Source: CAD feature listing. Evaluate the final solid. Frame: model axes, mm. Face numbers are marked on the shaded views. Round coordinates to 2 decimals unless told otherwise and drop trailing zeros. Loops run counter-clockwise (first coordinate to the right, second up) from the corner with the lowest first, then second, coordinate; pieces in that order, holes last. Notation, with made-up numbers: M -33.5,-22.5 L -1.5,-22.5 A6 cw -1.5,-18.5 Z; hole C -21,-15 d7. An arc over 180 degrees is marked long. Answer as CSV lines item,"result". Start each with the question number.
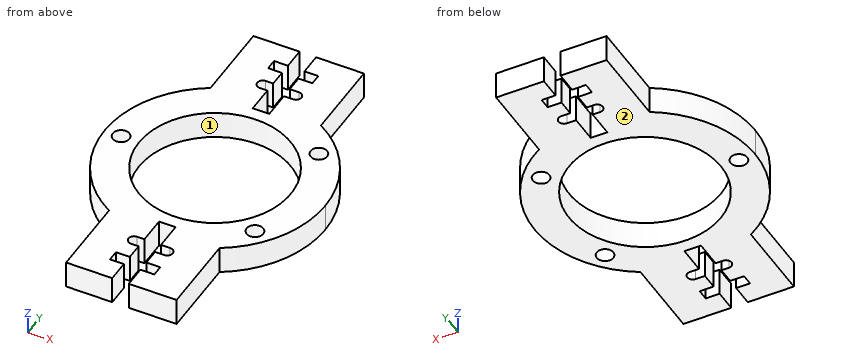
```python
from build123d import *
from build123d.topology import SkipClean

# Parameters (mm, degrees)
SKETCH1_R           = 1.5
BOSS_EXTRUDE1_DEPTH = 5


with BuildPart() as part:
    # Sketch1 → Boss-Extrude1 (new body)
    with BuildSketch(Plane(origin=(0, 0, 0), x_dir=(-0.9999998655639977, -0.000518528674721734, 0), z_dir=(0, 0, 1))):
        with BuildLine():
            Line((20, 0), (18.5, 0))
            ThreePointArc((18.5, 0), (17, -1.5), (15.5, 0))
            Line((15.5, 0), (13.75, 0))
            ThreePointArc((13.75, 0), (0, -13.75), (-13.75, 0))
            Line((-13.75, 0), (-20, 0))
            ThreePointArc((-20, 0), (-17.320508076, -10), (-10, -17.320508076))
            Line((-10, -17.320508076), (-10, -32))
            Line((-10, -32), (-1.347069158, -32))
            Line((-1.347069158, -32), (-1.347069158, -28.031929013))
            Line((-1.347069158, -28.031929013), (-3.861161574, -28.031929013))
            Line((-3.861161574, -28.031929013), (-3.861161574, -26))
            Line((-3.861161574, -26), (-1.347069158, -26))
            Line((-1.347069158, -26), (-1.347069158, -23))
            Line((-1.347069158, -23), (-3, -23))
            ThreePointArc((-3, -23), (-4, -22), (-3, -21))
            Line((-3, -21), (-1.347069158, -21))
            Line((-1.347069158, -21), (-1.347069158, -16))
            Line((-1.347069158, -16), (1.652930842, -16))
            Line((1.652930842, -16), (1.652930842, -21))
            Line((1.652930842, -21), (3, -21))
            ThreePointArc((3, -21), (4, -22), (3, -23))
            Line((3, -23), (1.652930842, -23))
            Line((1.652930842, -23), (1.652930842, -26))
            Line((1.652930842, -26), (4.167023259, -26))
            Line((4.167023259, -26), (4.167023259, -28.031929013))
            Line((4.167023259, -28.031929013), (1.652930842, -28.031929013))
            Line((1.652930842, -28.031929013), (1.652930842, -32))
            Line((1.652930842, -32), (10, -32))
            Line((10, -32), (10, -17.320508076))
            ThreePointArc((10, -17.320508076), (17.320508076, -10), (20, 0))
        make_face()
        with Locations(Location((-13.022755533, -10.927389365, 0), (0, 0, 179.970290494))):
            Circle(SKETCH1_R, mode=Mode.SUBTRACT)
    boss_extrude1 = extrude(amount=BOSS_EXTRUDE1_DEPTH)

    # Mirror1: Boss-Extrude1 across plane
    with SkipClean():  # the faces are left unmerged after this step: merging them gives an invalid solid
        add(boss_extrude1.mirror(Plane(origin=(-1.06692597, -0.000553232, 5), x_dir=(0, 0, 1), z_dir=(-0.0005185286747217338, 0.9999998655639978, 0))))


solid = part.part
```
1) Section C-C, the plane x = -8.5. Return loops of the section in (y, z).
2) Section D-D, the plane z = 1.3. Give the number of separate pieces and of enclosed holes in the cut face, and give its area (3 significant figures).
3) Section B-B, the plane x = 13. Return loops of the section in (y, z).
4) Ray query, line 1 along X through (y, z) = (0, 1.75); line 2 along X through (y, z) = (-26.5, 1.35); line 3 along X through (y, z) = (25, 2.9). Return the intervals inside material, ascending.
5) Section A-A, the plane x = 0. Return loops of the section in (y, z), and give its area (3 significant figures).
6) Contact query for flat-ended pins moving along their axis: pin 1 Ø1.8 at (x, y) = (-17, -0.01) entering from -Z; pin 2 Ø2 at (x, z) = (-13.5, 2) entering from -Y; pin 3 Ø1.5 at (y, z) = (6, 1) entering from +X; pin 4 Ø2 at (y, z) = (24, 3.5) entering from +X. Output: stop coordinate, or through.
7) Mould query, pull axis X, two halves, no side actions, for the marked faces 1 and 2. Classes: pulls with the +X half, pulls with the -X half, needs draft (parallel to the pull), parting line crosses it, or undercut.
Findings below:
1,outline,"M -32,0 L -10.81,0 L -10.81,5 L -32,5 Z; M 10.81,0 L 32,0 L 32,5 L 10.81,5 Z"
2,separate pieces,"1"
2,enclosed holes,"4"
2,area,"1,020 mm²"
3,outline,"M -15.2,0 L -12.42,0 L -12.42,5 L -15.2,5 Z; M -9.42,0 L -4.48,0 L -4.48,5 L -9.42,5 Z; M 4.48,0 L 9.43,0 L 9.43,5 L 4.48,5 Z; M 12.43,0 L 15.2,0 L 15.2,5 L 12.43,5 Z"
4,line 1,"-20 to -18.5, -15.5 to -13.75, 13.75 to 20"
4,line 2,"-9.99 to -4.15, 3.87 to 10.01"
4,line 3,"-10.01 to -1.67, 1.33 to 9.99"
5,outline,"M -16,0 L -13.75,0 L -13.75,5 L -16,5 Z; M 13.75,0 L 16,0 L 16,5 L 13.75,5 Z"
5,area,"22.5 mm²"
6,pin 1,"through"
6,pin 2,"y = -15.61"
6,pin 3,"x = 19.3"
6,pin 4,"x = 9.99"
7,face 1,"undercut"
7,face 2,"needs draft"
